Build history of the part. All positions in model axes, mm. A direction names the side the tool comes from. Coordinates: 2 decimals unless noted, no trailing zeros. Write each loop counter-clockwise with the first axis right and the second up, starting at its lowest first coordinate (ties: lowest second). Pieces come first, ordered by that corner, then holes.
```python
from build123d import *

# Parameters (mm, degrees)
SKETCH2_R           = 2.95
SKETCH2_R_2         = 1.975
SKETCH2_W           = 5
SKETCH2_H           = 5
BOSS_EXTRUDE1_DEPTH = 5


with BuildPart() as part:
    # Sketch2 → Boss-Extrude1 (new body)
    with BuildSketch(Plane.XY):
        Polygon((66.5, 15), (70, 15), (70, 20), (75, 20), (75, 15), (80, 15), (80, -15), (75, -15), (75, -20), (70, -20), (70, -15), (66.5, -15), (66.5, -12), (67.6, -12), (67.6, -9.7), (66.5, -9.7), (66.5, -5), (63.5, -5), (63.5, -9.7), (62.4, -9.7), (62.4, -12), (63.5, -12), (63.5, -15), (60, -15), (60, -20), (55, -20), (55, -15), (-55, -15), (-55, -20), (-60, -20), (-60, -15), (-63.5, -15), (-63.5, -12), (-62.4, -12), (-62.4, -9.7), (-63.5, -9.7), (-63.5, -5), (-66.5, -5), (-66.5, -9.7), (-67.6, -9.7), (-67.6, -12), (-66.5, -12), (-66.5, -15), (-70, -15), (-70, -20), (-75, -20), (-75, -15), (-80, -15), (-80, 15), (-75, 15), (-75, 20), (-70, 20), (-70, 15), (-66.5, 15), (-66.5, 12), (-67.6, 12), (-67.6, 9.7), (-66.5, 9.7), (-66.5, 5), (-63.5, 5), (-63.5, 9.7), (-62.4, 9.7), (-62.4, 12), (-63.5, 12), (-63.5, 15), (-60, 15), (-60, 20), (-55, 20), (-55, 15), (55, 15), (55, 20), (60, 20), (60, 15), (63.5, 15), (63.5, 12), (62.4, 12), (62.4, 9.7), (63.5, 9.7), (63.5, 5), (66.5, 5), (66.5, 9.7), (67.6, 9.7), (67.6, 12), (66.5, 12), align=None)
        with Locations((23.25, 0)):
            Circle(SKETCH2_R, mode=Mode.SUBTRACT)
        with Locations(Location((16.75, 0, 0), (0, 0, 180))):
            Circle(SKETCH2_R, mode=Mode.SUBTRACT)
        with Locations((38.25, 0)):
            Circle(SKETCH2_R_2, mode=Mode.SUBTRACT)
        with Locations((-52.5, 7.5)):
            Rectangle(SKETCH2_W, SKETCH2_H, mode=Mode.SUBTRACT)
        with Locations((-52.5, -7.5)):
            Rectangle(SKETCH2_W, SKETCH2_H, mode=Mode.SUBTRACT)
        with Locations((52.5, 7.5)):
            Rectangle(SKETCH2_W, SKETCH2_H, mode=Mode.SUBTRACT)
        with Locations((52.5, -7.5)):
            Rectangle(SKETCH2_W, SKETCH2_H, mode=Mode.SUBTRACT)
    extrude(amount=BOSS_EXTRUDE1_DEPTH)


solid = part.part
```
1. 3-axis set-ups, long thin cutter, end or side, ignore diameter. For faces 1 (the face through (50, 7, 2)), 2 (the face through (62, 15, 2)), 3 (the face through (78, -15, 2)), 4 (the face through (-75, 17, 2)), 5 (the face through (-66.5, -13, 2)): which of +Z, -Z, +X, -X, +Y, -Y reach the whole face in a straight line?
Computed values:
face 1: +Z, -Z
face 2: +Z, -Z, +Y
face 3: +Z, -Z, +X, -Y
face 4: +Z, -Z, -X, +Y
face 5: +Z, -Z, -Y
2. Mould opens along Y. For faces 6 (the face through (-55, 7, 2)), 7 (the face through (-63.5, 7, 2)), 8 (the face through (77, 15, 2)) say: +Y half, -Y half, draft (parallel to the pull), parting line (faces both ways), or undercut.
Computed values:
face 6: undercut
face 7: draft
face 8: +Y half
3. Saw through at A-A on x = 16.75. List the corners of the cut face in (y, z).
Computed values:
outline: (-15, 0) - (-2.95, 0) - (-2.95, 5) - (-15, 5) - close; (2.95, 0) - (15, 0) - (15, 5) - (2.95, 5) - close
4. Saw through at D-D on z = 2.3. State how many separate pieces and enclosed holes the cut face has, plus the area to 3 significant figures.
Computed values:
separate pieces: 1
enclosed holes: 7
area: 4,690 mm2
5. Saw through at B-B on y = 0. List the corners of the cut face in (x, z) (3 decimals), plus the area to 3 significant figures.
Computed values:
outline: (-80, 0) - (13.8, 0) - (13.8, 5) - (-80, 5) - close; (19.7, 0) - (20.3, 0) - (20.3, 5) - (19.7, 5) - close; (26.2, 0) - (36.275, 0) - (36.275, 5) - (26.2, 5) - close; (40.225, 0) - (80, 0) - (80, 5) - (40.225, 5) - close
area: 721 mm2
6. Saw through at C-C on x = 38.25. List the corners of the cut face in (y, z) (3 decimals).
Computed values:
outline: (-15, 0) - (-1.975, 0) - (-1.975, 5) - (-15, 5) - close; (1.975, 0) - (15, 0) - (15, 5) - (1.975, 5) - close
7. Flat gauge pins, fed straight in: pin 1 (10 mm diameter, centred on x = 16.5, y = -12.5, fed in from -Z); pin 2 (1.2 mm diameter, centred on x = -67, z = 3.5, fed in from +Y); pin 3 (1.5 mm diameter, centred on y = 18, z = 2, fed in from +X); pin 4 (1.5 mm diameter, centred on x = -76.5, z = 2.5, fed in from -Y). Where does each tip first touch, or does it go through?
Computed values:
pin 1: stops at z = 0
pin 2: stops at y = 15
pin 3: stops at x = 75
pin 4: stops at y = -15
8. Probe line 1 along X through (y, z) = (7, 2.75); line 2 along Y through (x, z) = (-52.5, 4); line 3 along X through (y, z) = (-14, 4.4). List the from-to ranges inside material, lowest first.
Computed values:
line 1: x = -80 to -66.5, -63.5 to -55, -50 to 50, 55 to 63.5, 66.5 to 80
line 2: y = -15 to -10, -5 to 5, 10 to 15
line 3: x = -80 to -66.5, -63.5 to 63.5, 66.5 to 80
